Source: three-view drawing plus pictorial views. Frame: mm from the lowest corner of the part. A direction names the side the tool comes from. Give positions to 0.01 mm unless a question says otherwise; leave off trailing zeros. Loops run counter-clockwise (first coordinate to the right, second up) from the corner with the lowest first, then second, coordinate; pieces in that order, holes last. Notation, with made-up numbers: M 9.5,-28 L 47.5,-28 A20 cw 47.5,-13 Z; hole C 83,-33 d9. An arc over 180 degrees is marked long. Answer as a JSON object with one key per item and string values. Group by question number.
1) Section query A-A on y = 11.25. Return loops of the section in (x, z), plus the area to 3 significant figures.
2) Access query for the marked faces 1 and 2. Directions: +Z, -Z, +X, -X, +Y, -Y. A direction counts if a zero-diameter tool reaches every point of the face in a straight line with its end or side. Return the directions, or none.
3) Ray query, L1, parallel to Y at x = 10, z = 134.5; L2, parallel to Z at x = 10.75, y = 1; L3, parallel to Y at x = 4.5, z = 141. Return the intervals inside material, ascending.
4) First-contact query: P1, Ø3, axis at x = 10, z = 178.5, coming from the -Y side; P2, Ø10, axis at x = 7, y = 3.5, coming from the +Z side; P3, Ø10, axis at y = 7.5, z = 189.5, coming from the +X side; P4, Ø10, axis at y = 18.5, z = 24, coming from the -X side. Flat tips, straight axial feed; report the tip coordinate or a pass-through.
5) Section query B-B on x = 10. Return loops of the section in (y, z).
6) Section query C-C on z = 189.5. Return loops of the section in (x, y).
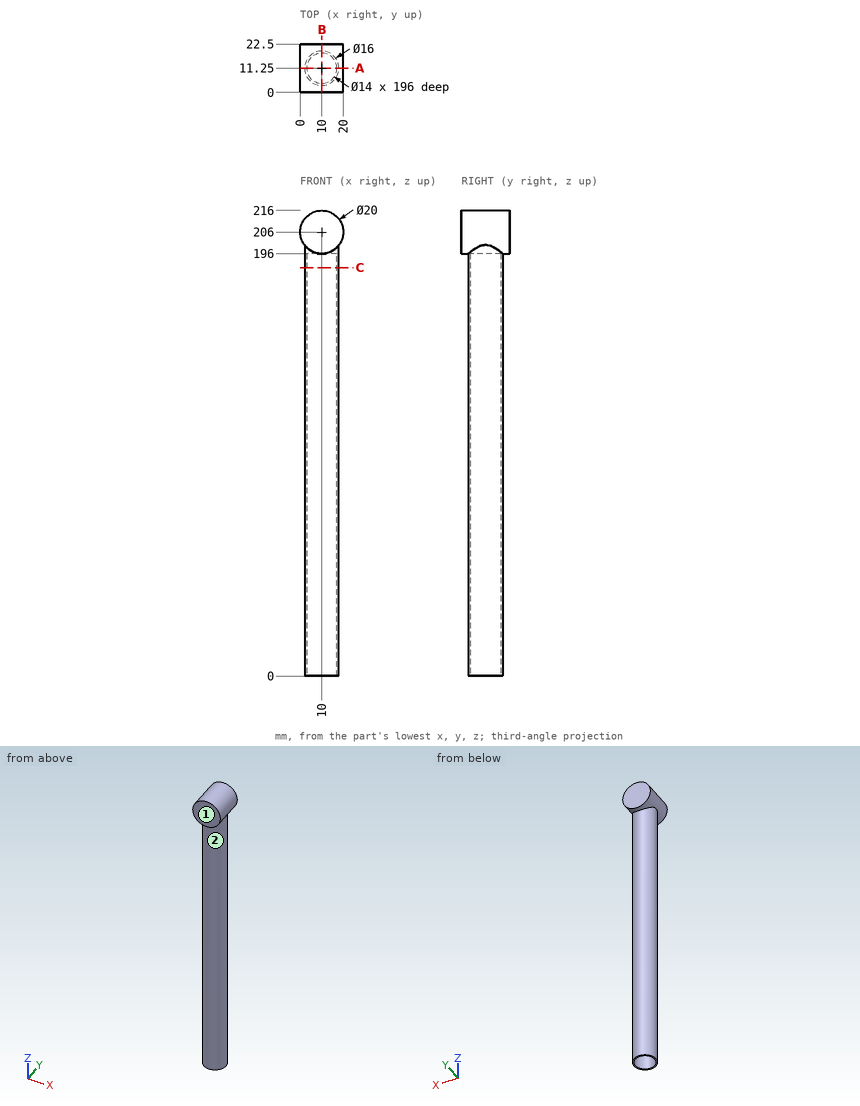
Output:
{
 "1": {"outline": "M 2,0 L 3,0 L 3,196 L 17,196 L 17,0 L 18,0 L 18,200 A10 ccw long 2,200 Z", "area": "725 mm^2"},
 "2": {"face 1": "+Z, -Z, +X, -X, -Y", "face 2": "-Z"},
 "3": {"L1": "y = 3.25 to 4.25, 18.25 to 19.25", "L2": "z = 196.03 to 215.97", "L3": "y = 5.44 to 6.92, 15.58 to 17.06"},
 "4": {"P1": "stops at y = 3.25", "P2": "stops at z = 216", "P3": "stops at x = 18", "P4": "stops at x = 2.32"},
 "5": {"outline": "M 0,196 L 3.25,196 L 3.25,0 L 4.25,0 L 4.25,196 L 18.25,196 L 18.25,0 L 19.25,0 L 19.25,196 L 22.5,196 L 22.5,216 L 0,216 Z"},
 "6": {"outline": "C 10,11.25 d16; hole C 10,11.25 d14"}
}
